```python
from build123d import *

# Parameters (mm, degrees)
F0_R     = 0.9
F0_R_2   = 0.95
F0_R_3   = 1
F0_R_4   = 1.05
F0_R_5   = 1.1
F1_DEPTH = 3.125


with BuildPart() as f1:
    # F0 (on Top) → F1 (new body)
    with BuildSketch(Plane.XY):
        with BuildLine():
            Line((-12.1, -5.1), (12.1, -5.1))
            ThreePointArc((12.1, -5.1), (12.807107, -4.807107), (13.1, -4.1))
            Line((13.1, -4.1), (13.1, 4.1))
            ThreePointArc((13.1, 4.1), (12.807107, 4.807107), (12.1, 5.1))
            Line((12.1, 5.1), (-12.1, 5.1))
            ThreePointArc((-12.1, 5.1), (-12.807107, 4.807107), (-13.1, 4.1))
            Line((-13.1, 4.1), (-13.1, -4.1))
            ThreePointArc((-13.1, -4.1), (-12.807107, -4.807107), (-12.1, -5.1))
        make_face()
        with Locations((-8, 0)):
            Circle(F0_R, mode=Mode.SUBTRACT)
        with Locations((-4, 0)):
            Circle(F0_R_2, mode=Mode.SUBTRACT)
        Circle(F0_R_3, mode=Mode.SUBTRACT)
        with Locations((4, 0)):
            Circle(F0_R_4, mode=Mode.SUBTRACT)
        with Locations((8, 0)):
            Circle(F0_R_5, mode=Mode.SUBTRACT)
    extrude(amount=F1_DEPTH)


solid = f1.part
```
Here's how the part is built. I have some questions about the finished solid (model axes, mm). Give positions to 0.01 mm unless a question says otherwise; leave off trailing zeros. Loops run counter-clockwise (first coordinate to the right, second up) from the corner with the lowest first, then second, coordinate; pieces in that order, holes last. Notation, with made-up numbers: M 73.25,-29 L 90.25,-29 A27 cw 90.25,-7 Z; hole C 80.5,33.25 d8. An arc over 180 degrees is marked long. Return JSON: item names as keys, results as strings.
Item 1: Imagine slicing it at A-A on y = 0. List the corners of the cut face in (x, z) for me (3 decimals), then the cut area to 3 significant figures.
A:
{"outline": "M -13.1,0 L -8.9,0 L -8.9,3.125 L -13.1,3.125 Z; M -7.1,0 L -4.95,0 L -4.95,3.125 L -7.1,3.125 Z; M -3.05,0 L -1,0 L -1,3.125 L -3.05,3.125 Z; M 1,0 L 2.95,0 L 2.95,3.125 L 1,3.125 Z; M 5.05,0 L 6.9,0 L 6.9,3.125 L 5.05,3.125 Z; M 9.1,0 L 13.1,0 L 13.1,3.125 L 9.1,3.125 Z", "area": "50.6 mm^2"}
Item 2: Imagine slicing it at D-D on x = 4. List the corners of the cut face in (y, z) for me (3 decimals), then the cut area to 3 significant figures.
A:
{"outline": "M -5.1,0 L -1.05,0 L -1.05,3.125 L -5.1,3.125 Z; M 1.05,0 L 5.1,0 L 5.1,3.125 L 1.05,3.125 Z", "area": "25.3 mm^2"}
Item 3: Thinking about a two-plate mould opening in X: for faces 1 (the cylindrical face through (-12.799, 4.815, 1.541)), 2 (the flat face through (-0.2, 1.2, 0)), 3 (the cylindrical face through (-4.95, 0.04, 1.54)), which applies, released by +X, released by -X, zero draft, split by the parting line, or undercut?
A:
{"face 1": "released by -X", "face 2": "zero draft", "face 3": "undercut"}
Item 4: Imagine slicing it at C-C on z = 2.1. List the corners of the cut face in (x, y) for me.
A:
{"outline": "M -13.1,-4.1 A1 ccw -12.1,-5.1 L 12.1,-5.1 A1 ccw 13.1,-4.1 L 13.1,4.1 A1 ccw 12.1,5.1 L -12.1,5.1 A1 ccw -13.1,4.1 Z; hole C -8,0 d1.8; hole C -4,0 d1.9; hole C 0,0 d2; hole C 4,0 d2.1; hole C 8,0 d2.2"}
Item 5: Please list where these lines run through material, in increasing order: line 1 (Y direction, x = 8, z = 1.6); line 2 (Y direction, x = -8, z = 0.2).
A:
{"line 1": "y = -5.1 to -1.1, 1.1 to 5.1", "line 2": "y = -5.1 to -0.9, 0.9 to 5.1"}
Item 6: Imagine slicing it at B-B on x = 8. List the corners of the cut face in (y, z) for me (3 decimals).
A:
{"outline": "M -5.1,0 L -1.1,0 L -1.1,3.125 L -5.1,3.125 Z; M 1.1,0 L 5.1,0 L 5.1,3.125 L 1.1,3.125 Z"}
